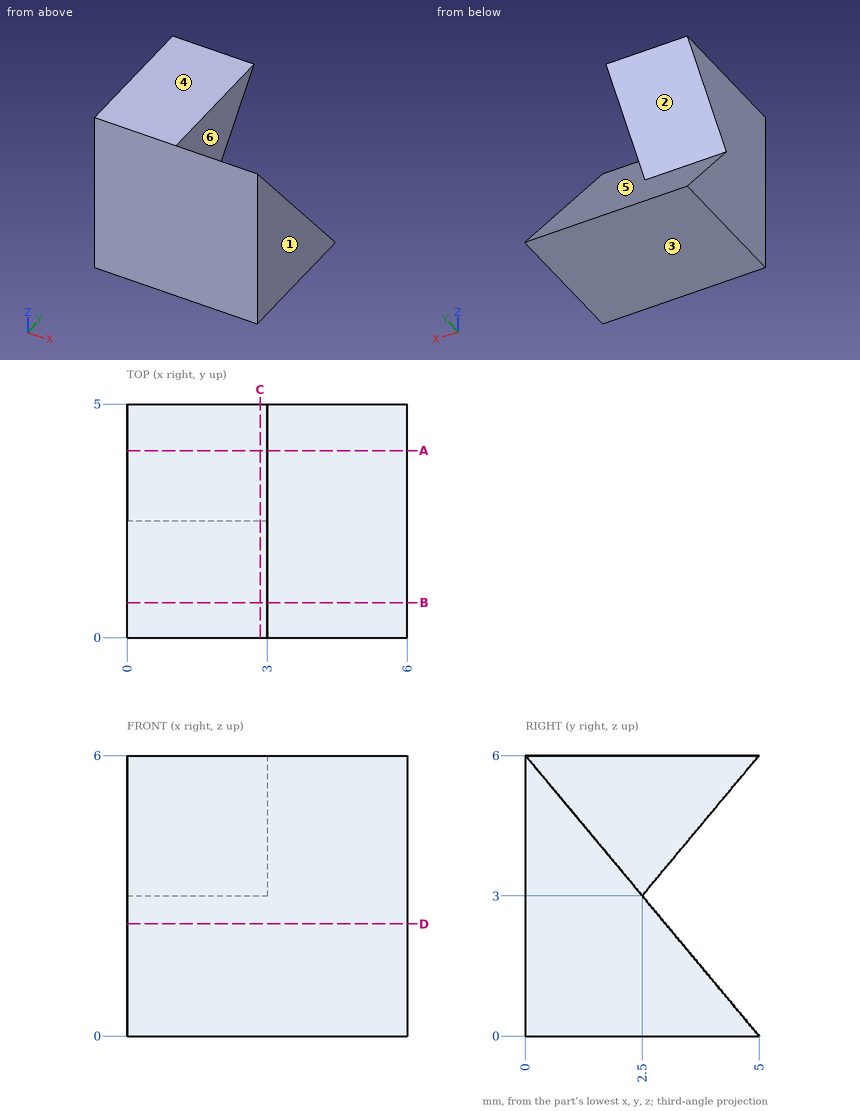
Here's the drawing with two shaded views (mm, measured from the low corner). I have some questions. A direction names the side the tool comes from. Give positions to 0.01 mm unless a question says otherwise; leave off trailing zeros. Order: outer loops, then holes, each group sorted by start corner. A loop starts at its lowest first (then second) coordinate and runs counter-clockwise, first axis right, second up. Notation, with made-up numbers: M 83,-20.75 L 141,-20.75 A12 ccw 141,-15.75 Z; hole C 41,-17.5 d8. An arc over 180 degrees is marked long. One line per item, written item: value.
1) For P1, Ø2, axis at x = 1, z = 0.5, coming from the +Y side; P2, Ø2, axis at x = 4.5, z = 3, coming from the +Y side, each with a flat end and sliding along its axis, tell me the tip position at first contact or that it passes through.
Answer sheet:
P1: stops at y = 5
P2: stops at y = 3.33
2) I want a section at D-D, the plane z = 2.4. List the corners of the cut face in (x, y) for me, plus the area to 3 significant figures.
Answer sheet:
outline: M 0,0 L 6,0 L 6,3 L 0,3 Z
area: 18.0 mm^2
3) We'd pull the mould along Z, two halves only. Please class the marked faces 3, 4, 5 and 6: released by +Z, released by -Z, zero draft, split by the parting line, or undercut.
Answer sheet:
face 3: released by -Z
face 4: released by +Z
face 5: undercut
face 6: zero draft
4) On a 3-axis mill with a long thin cutter (end or side, diameter ignored), from which of +Z, -Z, +X, -X, +Y, -Y can I reach the whole of each face in a straight line? I mean the marked faces 1 and 2. Say none if no direction works.
Answer sheet:
face 1: +Z, -Z, +X, +Y, -Y
face 2: +X, -X, +Y
5) I want a section at B-B, the plane y = 0.75. List the corners of the cut face in (x, z) for me.
Answer sheet:
outline: M 0,0 L 6,0 L 6,5.1 L 3,5.1 L 3,6 L 0,6 Z
6) Please list where these lines run through material, in increasing order: line 1 along X through (y, z) = (4, 5.1); line 2 along Z through (x, y) = (1.45, 4.6); line 3 along Z through (x, y) = (3.8, 1.9).
Answer sheet:
line 1: x = 0 to 3
line 2: z = 0 to 0.48, 5.52 to 6
line 3: z = 0 to 3.72
7) I want a section at A-A, the plane y = 4. List the corners of the cut face in (x, z) for me.
Answer sheet:
outline: M 0,0 L 6,0 L 6,1.2 L 0,1.2 Z; M 0,4.8 L 3,4.8 L 3,6 L 0,6 Z
8) I want a section at C-C, the plane x = 2.85. List the corners of the cut face in (y, z) for me, plus the area to 3 significant figures.
Answer sheet:
outline: M 0,0 L 5,0 L 2.5,3 L 5,6 L 0,6 Z
area: 22.5 mm^2
